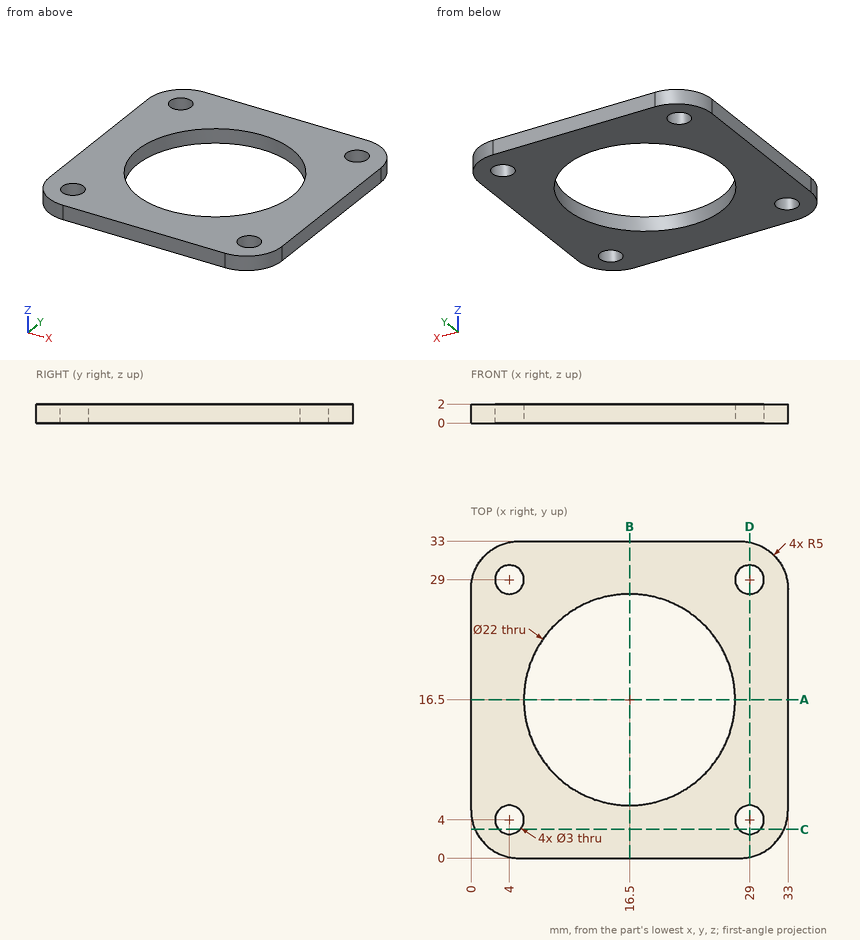
Check sheet for the drawn part. Datum: minimum x, y, z corner. Units: mm. Give positions to 0.01 mm unless a question says otherwise; leave off trailing zeros. Loops run counter-clockwise (first coordinate to the right, second up) from the corner with the lowest first, then second, coordinate; pieces in that order, holes last. Notation, with made-up numbers: M -27.5,-13 L 5.5,-13 A27 cw 5.5,15 Z; hole C 3.25,33.25 d1. An arc over 180 degrees is marked long. Return JSON: item names as keys, results as strings.
1) Section check A-A, the plane y = 16.5. Enter the section's corners in (x, z), and give its area (3 significant figures).
Findings:
{"outline": "M 0,0 L 5.5,0 L 5.5,2 L 0,2 Z; M 27.5,0 L 33,0 L 33,2 L 27.5,2 Z", "area": "22.0 mm2"}
2) Section check C-C, the plane y = 3. Enter the section's corners in (x, z), and give its area (3 significant figures).
Findings:
{"outline": "M 0.42,0 L 2.88,0 L 2.88,2 L 0.42,2 Z; M 5.12,0 L 27.88,0 L 27.88,2 L 5.12,2 Z; M 30.12,0 L 32.58,0 L 32.58,2 L 30.12,2 Z", "area": "55.4 mm2"}
3) Material ranges on L1, parallel to Y at x = 4, z = 1.3; L2, parallel to X at y = 3.5, z = 0.9; L3, parallel to X at y = 3, z = 0.5, recorded low to high. Write a range as [from, to].
Findings:
{"L1": "y = [0.1, 2.5], [5.5, 27.5], [30.5, 32.9]", "L2": "x = [0.23, 2.59], [5.41, 27.59], [30.41, 32.77]", "L3": "x = [0.42, 2.88], [5.12, 27.88], [30.12, 32.58]"}
4) Section check D-D, the plane x = 29. Enter the section's corners in (y, z).
Findings:
{"outline": "M 0.1,0 L 2.5,0 L 2.5,2 L 0.1,2 Z; M 5.5,0 L 27.5,0 L 27.5,2 L 5.5,2 Z; M 30.5,0 L 32.9,0 L 32.9,2 L 30.5,2 Z"}
